from build123d import *

# Parameters (mm, degrees)
ESBO_O1_R                = 1.5
ESBO_O1_W                = 20
ESBO_O1_H                = 8
ESBO_O1_W_2              = 15
ESBO_O1_H_2              = 7.5
RESSALTO_EXTRUS_O1_DEPTH = 4
CORTE_EXTRUS_O1_DEPTH    = 10
FILETE1_R                = 2
ESBO_O3_R                = 1.25
CORTE_EXTRUS_O2_DEPTH    = 12


with BuildPart() as part:
    # Esboço1 → Ressalto-extrusão1 (new body)
    with BuildSketch(Plane.XY):
        Polygon((0, 0), (96.01, 0), (96.01, -58), (75.01, -58), (75.01, -66), (96.01, -66), (96.01, -70), (0, -70), (0, -66), (21, -66), (21, -58), (0, -58), align=None)
        with Locations((48.005, -25)):
            Circle(ESBO_O1_R, mode=Mode.SUBTRACT)
        with Locations((86.01, -25)):
            Circle(ESBO_O1_R, mode=Mode.SUBTRACT)
        with Locations((10, -25)):
            Circle(ESBO_O1_R, mode=Mode.SUBTRACT)
        with Locations((66.01, -25)):
            Circle(ESBO_O1_R, mode=Mode.SUBTRACT)
        with Locations((30, -25)):
            Circle(ESBO_O1_R, mode=Mode.SUBTRACT)
        with Locations((48.005, -62)):
            Rectangle(ESBO_O1_W, ESBO_O1_H, mode=Mode.SUBTRACT)
        with Locations((48.005, -36.75)):
            Rectangle(ESBO_O1_W_2, ESBO_O1_H_2, mode=Mode.SUBTRACT)
    extrude(amount=RESSALTO_EXTRUS_O1_DEPTH)

    # Esboço2 → Corte-extrusão1 (cut)
    with BuildSketch(Plane.XY.offset(4)):
        Polygon((63.01, -39.351037912), (81.01, -39.351037912), (72.01, -54.93949518), align=None)
        Polygon((15, -39.351037912), (33, -39.351037912), (24, -54.93949518), align=None)
    extrude(amount=-CORTE_EXTRUS_O1_DEPTH, mode=Mode.SUBTRACT)

    # Filete1
    filete1_edges = [part.edges().sort_by_distance(p)[0] for p in [
        (72.01, -54.93949518, 2),
        (63.01, -39.351037912, 2),
        (81.01, -39.351037912, 2),
        (24, -54.93949518, 2),
        (15, -39.351037912, 2),
        (33, -39.351037912, 2),
    ]]
    fillet(filete1_edges, radius=FILETE1_R)

    # Esboço3 → Corte-extrusão2 (cut)
    with BuildSketch(Plane.XZ.offset(70)):
        with Locations((25, 2)):
            Circle(ESBO_O3_R)
        with Locations((34, 2)):
            Circle(ESBO_O3_R)
        with Locations((62.01, 2)):
            Circle(ESBO_O3_R)
        with Locations((71.01, 2)):
            Circle(ESBO_O3_R)
    extrude(amount=-CORTE_EXTRUS_O2_DEPTH, mode=Mode.SUBTRACT)


solid = part.part
Read the model definition and answer for the solid it produces. Units are mm, in the model's axes. A direction names the side the tool comes from. Round coordinates to 2 decimals unless told otherwise and drop trailing zeros. Order: outer loops, then holes, each group sorted by start corner. A loop starts at its lowest first (then second) coordinate and runs counter-clockwise, first axis right, second up. Notation, with made-up numbers: (40, 18) - (58, 18) arc R13 cw to (58, 36) - close; hole circle Ø11 at (-6, 78). An arc over 180 degrees is marked (long way). Use one line per item in the form item = value. Start each with the question number.
(1) The part is cut by section C-C (x = 62.01). Give the vertices of the cut face in (y, z), then the cut area to 3 significant figures.
(2) For faces 5 (the face through (86, -58, 2)), 6 (the face through (47, 0, 2)), 7 (the face through (58.005, -62, 2)), 8 (the face through (69.76, -64.08, 2.05)), determine the directions among +Z, -Z, +X, -X, +Y, -Y from which every point of the face is accessible in a straight line to the end or side of a thin tool.
(3) The part is cut by section D-D (z = 1.35). Count the separate pieces of the cut face and the enclosed holes in it, then the cut area to 3 significant figures.
(4) Determine the mould class of faces 1 (the face through (96.01, -68, 2)), 2 (the face through (24.03, -52.94, 1.97)), 3 (the face through (0, -68, 2)), 4 (the face through (49, -27, 0)) for opening direction X: +X half, -X half, draft (parallel to the pull), parting line (faces both ways), or undercut.
(5) Find the intervals of material crossed by line 1 along Y through (x, z) = (86, 1.8); line 2 along X through (y, z) = (-60.5, 3.1) (3 decimals); line 3 along Y through (x, z) = (81, 0.8), in increasing order. Write a range as from..to.
(6) Flat-ended cylindrical pins translate along their axes: pin 1 Ø0.8 at (x, z) = (34, 2) entering from -Y; pin 2 Ø2 at (y, z) = (-62, 1) entering from +X. Find the tip coordinate at first contact, or state that the pin passes through.
(7) The part is cut by section B-B (y = -49). Give the vertices of the cut face in (x, z).
(8) The part is cut by section A-A (x = 10). Give the vertices of the cut face in (y, z), then the cut area to 3 significant figures.
Checked values:
q1.outline = (-70, 0) - (0, 0) - (0, 4) - (-70, 4) - (-70, 3.25) - (-58, 3.25) - (-58, 0.75) - (-70, 0.75) - close
q1.area = 250 mm^2
q2.face_5 = +Z, -Z, +X
q2.face_6 = +Z, -Z, +X, -X, +Y
q2.face_7 = +Z, -Z
q2.face_8 = -Y
q3.separate_pieces = 1
q3.enclosed_holes = 9
q3.area = 5,710 mm^2
q4.face_1 = +X half
q4.face_2 = undercut
q4.face_3 = -X half
q4.face_4 = draft
q5.line_1 = -70..-66, -58..-26.5, -23.5..0
q5.line_2 = 21..24.406, 25.594..33.406, 34.594..38.005, 58.005..61.416, 62.604..70.416, 71.604..75.01
q5.line_3 = -70..-66, -58..0
q6.pin_1 = -58
q6.pin_2 = 75.01
q7.outline = (0, 0) - (20.57, 0) - (20.57, 4) - (0, 4) - close; (27.43, 0) - (68.58, 0) - (68.58, 4) - (27.43, 4) - close; (75.44, 0) - (96.01, 0) - (96.01, 4) - (75.44, 4) - close
q8.outline = (-70, 0) - (-66, 0) - (-66, 4) - (-70, 4) - close; (-58, 0) - (-26.5, 0) - (-26.5, 4) - (-58, 4) - close; (-23.5, 0) - (0, 0) - (0, 4) - (-23.5, 4) - close
q8.area = 236 mm^2
